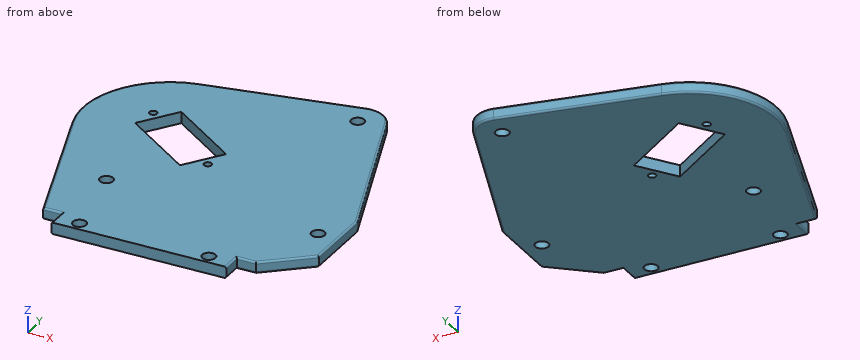
from build123d import *

# Parameters (mm, degrees)
SKETCH2_R               = 1
SKETCH2_R_2             = 1.75
BOSS_EXTRUDE1_DEPTH     = 1.5
FILLET1_R               = 0.5
FILLET2_R               = 0.5
CUT_EXTRUDE1_DEPTH      = 99.29192821
CUT_EXTRUDE1_DEPTH_BACK = 99.29192821
SKETCH3_W               = 46
SKETCH3_H               = 4.75


with BuildPart() as part:
    # Sketch2 → Boss-Extrude1 (new, symmetric)
    with BuildSketch(Plane.XY):
        with BuildLine():
            Line((39.405069621, 38.569989712), (22.934569539, 83.822316773))
            ThreePointArc((22.934569539, 83.822316773), (19.891485129, 87.41317775), (15.244648683, 88.162548371))
            Line((15.244648683, 88.162548371), (-24.631297069, 80.325625034))
            ThreePointArc((-24.631297069, 80.325625034), (-40.032912198, 69.313028262), (-41.860786126, 50.467712846))
            Line((-41.860786126, 50.467712846), (-28, 10))
            Line((-28, 10), (-23, 10))
            Line((-23, 10), (-23, 0))
            Line((-23, 0), (23, 0))
            Line((23, 0), (23, 10))
            Line((23, 10), (28, 10))
            Line((28, 10), (39.405069621, 19.569989712))
            Line((39.405069621, 19.569989712), (39.405069621, 38.569989712))
        make_face()
        with Locations((-27.182792376, 62.755399709)):
            Circle(SKETCH2_R, mode=Mode.SUBTRACT)
        with Locations((-4.246535136, 46.695259491)):
            Circle(SKETCH2_R, mode=Mode.SUBTRACT)
        with Locations((17, 7.4)):
            Circle(SKETCH2_R_2, mode=Mode.SUBTRACT)
        with Locations((-17, 7.4)):
            Circle(SKETCH2_R_2, mode=Mode.SUBTRACT)
        with Locations((34.155069621, 29.069989712)):
            Circle(SKETCH2_R_2, mode=Mode.SUBTRACT)
        with Locations((-21.5, 29.069989712)):
            Circle(SKETCH2_R_2, mode=Mode.SUBTRACT)
        with Locations((16.554056644, 81.5)):
            Circle(SKETCH2_R_2, mode=Mode.SUBTRACT)
        Polygon((-21.693453648, 66.236370884), (-28.576370884, 56.406546352), (-9.735873865, 43.214288316), (-2.852956629, 53.044112848), align=None, mode=Mode.SUBTRACT)
    extrude(amount=BOSS_EXTRUDE1_DEPTH, both=True)

    # Fillet1
    fillet1_edges = [part.edges().sort_by_distance(p)[0] for p in [
        (-40.032912198, 69.313028262, 1.5),
        (-34.930393063, 30.233856423, 1.5),
        (-25.5, 10, 1.5),
        (-23, 5, 1.5),
        (0, 0, 1.5),
        (23, 5, 1.5),
        (25.5, 10, 1.5),
        (33.70253481, 14.784994856, 1.5),
        (39.405069621, 29.069989712, 1.5),
        (31.16981958, 61.196153243, 1.5),
        (19.891485129, 87.41317775, 1.5),
        (-4.693324193, 84.244086702, 1.5),
    ]]
    fillet(fillet1_edges, radius=FILLET1_R)

    # Fillet2
    fillet2_edges = [part.edges().sort_by_distance(p)[0] for p in [
        (31.16981958, 61.196153243, -1.5),
        (39.405069621, 29.069989712, -1.5),
        (33.70253481, 14.784994856, -1.5),
        (25.5, 10, -1.5),
        (23, 5, -1.5),
        (0, 0, -1.5),
        (-23, 5, -1.5),
        (-25.5, 10, -1.5),
        (-34.930393063, 30.233856423, -1.5),
        (-40.032912198, 69.313028262, -1.5),
        (-4.693324193, 84.244086702, -1.5),
        (19.891485129, 87.41317775, -1.5),
    ]]
    fillet(fillet2_edges, radius=FILLET2_R)

    # Sketch3 → Cut-Extrude1 (cut, two sides: drawn at the far end of the back side and taken through both)
    with BuildSketch(Plane.XY.offset(1.5).offset(-CUT_EXTRUDE1_DEPTH_BACK)):
        with Locations((0, 2.375)):
            Rectangle(SKETCH3_W, SKETCH3_H)
    extrude(amount=CUT_EXTRUDE1_DEPTH + CUT_EXTRUDE1_DEPTH_BACK, mode=Mode.SUBTRACT)


solid = part.part
Geometry: final body of the model. Coordinates: model frame, mm. Give positions to 0.01 mm unless a question says otherwise; leave off trailing zeros. Write each loop counter-clockwise with the first axis right and the second up, starting at its lowest first coordinate (ties: lowest second). Pieces come first, ordered by that corner, then holes.
(1) Cut plane B-B, the plane z = -0.5. Give the number of separate pieces and of enclosed holes in the cut face, then the cut area to 3 significant figures.
(2) Ray query, line 1 (Y direction, x = 16.5, z = -1.3); line 2 (X direction, y = 51, z = -0.35); line 3 (Y direction, x = -14.5, z = -1.2). Return the intervals inside material, ascending.
(3) Cut plane A-A, the plane y = 7.4. Return loops of the section in (x, z).
(4) First-contact query: P1, Ø0.6, axis at y = 7.5, z = 0, coming from the +X side; P2, Ø4.5, axis at x = 16.55, y = 81.5, coming from the -Z side; P3, Ø0.6, axis at y = 6.5, z = 0, coming from the -X side; P4, Ø1, axis at x = -26.5, z = 0.5, coming from the -Y side. Flat tips, straight axial feed; report the tip coordinate or a pass-through.
Values follow:
1. separate pieces: 1
1. enclosed holes: 8
1. area: 5,120 mm2
2. line 1: y = 4.75 to 5.72, 9.08 to 79.75, 83.25 to 88.19
2. line 2: x = -42.04 to -20.86, -4.28 to 34.88
2. line 3: y = 4.75 to 46.55, 61.2 to 82.27
3. outline: (-23, -1) arc R0.5 ccw to (-22.5, -1.5) - (-18.75, -1.5) - (-18.75, 1.5) - (-22.5, 1.5) arc R0.5 ccw to (-23, 1) - close; (-15.25, -1.5) - (15.25, -1.5) - (15.25, 1.5) - (-15.25, 1.5) - close; (18.75, -1.5) - (22.5, -1.5) arc R0.5 ccw to (23, -1) - (23, 1) arc R0.5 ccw to (22.5, 1.5) - (18.75, 1.5) - close
4. P1: stops at x = 23
4. P2: stops at z = -1.5
4. P3: stops at x = -23
4. P4: stops at y = 10
